```python
from build123d import *

# Parameters (mm, degrees)
F0_R     = 2.5
F1_DEPTH = 5
F2_W     = 6.5
F2_H     = 3
F3_DEPTH = 25
F4_W     = 1.75
F4_H     = 1.75
F5_DEPTH = 3
F6_R     = 2.5
F7_DEPTH = 2.5


with BuildPart() as f1:
    # F0 (on Top) → F1 (new body)
    with BuildSketch(Plane.XY):
        with BuildLine():
            ThreePointArc((0, 4), (0.657671, 1.657671), (2.438447, 0))
            Line((2.438447, 0), (6.561553, 0))
            ThreePointArc((6.561553, 0), (8.342329, 1.657671), (9, 4))
            Line((9, 4), (7, 21))
            Line((7, 21), (7, 27.5))
            ThreePointArc((7, 27.5), (6.56066, 28.56066), (5.5, 29))
            Line((5.5, 29), (3.5, 29))
            ThreePointArc((3.5, 29), (2.43934, 28.56066), (2, 27.5))
            Line((2, 27.5), (2, 21))
            Line((2, 21), (0, 4))
        make_face()
        with Locations((4.5, 4)):
            Circle(F0_R, mode=Mode.SUBTRACT)
    extrude(amount=-F1_DEPTH)

    # F2 (on face) → F3 (cut)
    with BuildSketch(Plane.YZ.offset(7)):
        with Locations((24.25, -3.5)):
            Rectangle(F2_W, F2_H)
    extrude(amount=-F3_DEPTH, mode=Mode.SUBTRACT)

    # F4 (on face) → F5 (join, through all)
    with BuildSketch(Plane(origin=(0, 0, -2), x_dir=(1, 0, 0), z_dir=(0, 0, -1))):
        with Locations((4.5, -26.625)):
            Rectangle(F4_W, F4_H)
    extrude(amount=F5_DEPTH)

    # F6 (on face) → F7 (cut)
    with BuildSketch(Plane(origin=(0, 0, -5), x_dir=(1, 0, 0), z_dir=(0, 0, -1))):
        with BuildLine():
            ThreePointArc((2.438447, 0), (0.657671, -1.657671), (0, -4))
            Line((0, -4), (0.941176, -12))
            Line((0.941176, -12), (8.058824, -12))
            Line((8.058824, -12), (9, -4))
            ThreePointArc((9, -4), (8.342329, -1.657671), (6.561553, 0))
            Line((6.561553, 0), (2.438447, 0))
        make_face()
        with Locations((4.5, -4)):
            Circle(F6_R, mode=Mode.SUBTRACT)
    extrude(amount=-F7_DEPTH, mode=Mode.SUBTRACT)


solid = f1.part
```
Geometry: final body of the model. Coordinates: model frame, mm. A direction names the side the tool comes from. Give positions to 0.01 mm unless a question says otherwise; leave off trailing zeros. Write each loop counter-clockwise with the first axis right and the second up, starting at its lowest first coordinate (ties: lowest second). Pieces come first, ordered by that corner, then holes.
1. Section query B-B, the plane z = -4.6. Return loops of the section in (x, y) (3 decimals), then the cut area to 3 significant figures.
2. Section query A-A, the plane x = 4.5. Return loops of the section in (y, z).
3. Pin query (flat end, axial travel): P1, Ø1.8, axis at x = 2.5, z = -4, coming from the -Y side; P2, Ø0.6, axis at y = 24, z = -1, coming from the -X side; P3, Ø0.9, axis at y = 26.5, z = -3, coming from the -X side (3 decimals). Return the tip coordinate at first contact, or that it passes through.
4. Line query: probe 1 along Y at (x, z) = (4.5, -1.15); probe 2 along Y at (x, z) = (4, -3.9); probe 3 along X at (y, z) = (4, -1.6). Output: solid intervals per line, ascending.
5. Draft query along X for faces 6 (the cylindrical face through (6.885, 4.751, -1.232)), 7 (the flat face through (1.236, 14.508, -1.909)), 8 (the flat face through (4, 17, -5)), 9 (the flat face through (7.79, 14.27, -1.91)). Return one class per face: released by +X, released by -X, zero draft, split by the parting line, or undercut.
6. Section query C-C, the plane y = 5. Return loops of the section in (x, z).
7. Section query D-D, the plane z = -0.75. Return loops of the section in (x, y).
8. Reachability of faces 1 (the flat face through (5.375, 27, -3)), 2 (the flat face through (4, 7, -2.5)), 3 (the flat face through (2, 24, -1)), 4 (the flat face through (3, 27.5, -4)), 5 (the flat face through (5, 21, -4)) from +Z, -Z, +X, -X, +Y, -Y: full face, straight path, thin tool, end or side. Return the list, or none.
Computed:
1. outline: (0.941, 12) - (8.059, 12) - (7, 21) - (2, 21) - close; (2, 27.5) - (3.625, 27.5) - (3.625, 25.75) - (5.375, 25.75) - (5.375, 27.5) - (7, 27.5) arc R1.5 ccw to (5.5, 29) - (3.5, 29) arc R1.5 ccw to start
1. area: 64.1 mm2
2. outline: (0, -2.5) - (1.5, -2.5) - (1.5, 0) - (0, 0) - close; (6.5, -2.5) - (12, -2.5) - (12, -5) - (21, -5) - (21, -2) - (25.75, -2) - (25.75, -5) - (29, -5) - (29, 0) - (6.5, 0) - close
3. P1: stops at y = 12
3. P2: stops at x = 2
3. P3: stops at x = 3.625
4. probe 1: y = 0 to 1.5, 6.5 to 29
4. probe 2: y = 12 to 21, 25.75 to 29
4. probe 3: x = 0 to 2, 7 to 9
5. face 6: undercut
5. face 7: released by -X
5. face 8: zero draft
5. face 9: released by +X
6. outline: (0.12, -2.5) - (2.21, -2.5) - (2.21, 0) - (0.12, 0) - close; (6.79, -2.5) - (8.88, -2.5) - (8.88, 0) - (6.79, 0) - close
7. outline: (0, 4) arc R4.5 ccw to (2.44, 0) - (6.56, 0) arc R4.5 ccw to (9, 4) - (7, 21) - (7, 27.5) arc R1.5 ccw to (5.5, 29) - (3.5, 29) arc R1.5 ccw to (2, 27.5) - (2, 21) - close; hole circle Ø5 at (4.5, 4)
8. face 1: -Z, +X
8. face 2: -Z, +X, -X, -Y
8. face 3: +Z, -Z, -X, +Y
8. face 4: -Z, -X
8. face 5: -Z, +X, -X
